```python
from build123d import *

# Parameters (mm, degrees)
F0_W     = 38.1
F0_H     = 38.1
F0_R     = 6.35
F1_DEPTH = 3.175
F2_W     = 38.1
F2_H     = 12.7
F3_DEPTH = 25.4
F4_W     = 38.1
F4_H     = 12.7
F5_DEPTH = 43.18
F6_R     = 3.175
F7_DEPTH = 81.281


with BuildPart() as f1:
    # F0 (on Top) → F1 (new body)
    with BuildSketch(Plane.XY):
        with Locations((19.05, 19.05)):
            Rectangle(F0_W, F0_H)
        with Locations((19.05, 25.4)):
            Circle(F0_R, mode=Mode.SUBTRACT)
    extrude(amount=F1_DEPTH)

    # F2 (on face) → F3 (join)
    with BuildSketch(Plane.XY.offset(3.175)):
        with Locations((19.05, 6.35)):
            Rectangle(F2_W, F2_H)
    extrude(amount=F3_DEPTH)

    # F4 (on face) → F5 (join)
    with BuildSketch(Plane.XZ):
        with Locations((19.05, 22.225)):
            Rectangle(F4_W, F4_H)
    extrude(amount=F5_DEPTH)

    # F6 (on face) → F7 (cut, through all)
    with BuildSketch(Plane.XZ.offset(43.18)):
        with Locations((19.05, 22.225)):
            Circle(F6_R)
    extrude(amount=-F7_DEPTH, mode=Mode.SUBTRACT)


solid = f1.part
```
The listing builds one solid part. Answer for the finished solid, in the listing's coordinates (mm). A direction names the side the tool comes from. Give positions to 0.01 mm unless a question says otherwise; leave off trailing zeros. Write each loop counter-clockwise with the first axis right and the second up, starting at its lowest first coordinate (ties: lowest second). Pieces come first, ordered by that corner, then holes. Notation, with made-up numbers: (-12.75, 26) -> (37.25, 26) arc R21 ccw to (37.25, 54) -> close; hole circle Ø10 at (-4.75, 81.5). An arc over 180 degrees is marked (long way). Write item = value, one per line. Start each with the question number.
1) The part is cut by section D-D, the plane x = 34.5. Determine the outline of the cut face in (y, z) (3 decimals).
2) Determine the mould class of faces 1 (the face through (23, -43.18, 22)), 2 (the face through (38.1, -11, 17)), 3 (the face through (0, -11, 17)), 4 (the face through (24.916, 22.968, 1.565)) for opening direction X: +X half, -X half, draft (parallel to the pull), parting line (faces both ways), or undercut.
3) Each of these flat-tipped pins is pushed along its axis until it touches: pin 1 (12.5 mm diameter, centred on x = 19, z = 18, fed in from +Y); pin 2 (20.5 mm diameter, centred on x = 16.5, y = 31.5, fed in from +Z) (3 decimals); pin 3 (10 mm diameter, centred on x = 13, y = -22, fed in from -Z) (3 decimals). Where does it stop, or does it pass through?
4) The part is cut by section B-B, the plane y = 25.4. Determine the outline of the cut face in (x, z) (3 decimals).
5) Straight lines are drawn through the part: line 1 along Y through (x, z) = (19.05, 2.3); line 2 along Y through (x, z) = (36, 18.5); line 3 along Y through (x, z) = (27.5, 3.25). For each, find the intervals that lie inside material, in ascending order.
6) Which of the six approach directions +Z, -Z, +X, -X, +Y, -Y give full straight-line access (tool end or side, diameter ignored) to faces 5 (the face through (19, -15, 28.575)), 6 (the face through (19, 12.7, 16)), 7 (the face through (19, 0, 8))?
7) The part is cut by section C-C, the plane z = 23.75. Determine the outline of the cut face in (x, y).
8) The part is cut by section A-A, the plane x = 19.05. Determine the outline of the cut face in (y, z) (3 decimals).
Solutions:
q1.outline = (-43.18, 15.875) -> (0, 15.875) -> (0, 0) -> (38.1, 0) -> (38.1, 3.175) -> (12.7, 3.175) -> (12.7, 28.575) -> (-43.18, 28.575) -> close
q2.face_1 = draft
q2.face_2 = +X half
q2.face_3 = -X half
q2.face_4 = undercut
q3.pin_1 = 12.7
q3.pin_2 = 3.175
q3.pin_3 = 15.875
q4.outline = (0, 0) -> (12.7, 0) -> (12.7, 3.175) -> (0, 3.175) -> close; (25.4, 0) -> (38.1, 0) -> (38.1, 3.175) -> (25.4, 3.175) -> close
q5.line_1 = 0 to 19.05, 31.75 to 38.1
q5.line_2 = -43.18 to 12.7
q5.line_3 = 0 to 12.7
q6.face_5 = +Z, +X, -X, +Y, -Y
q6.face_6 = +Z, +X, -X, +Y
q6.face_7 = -Z, +X, -X, -Y
q7.outline = (0, -43.18) -> (16.27, -43.18) -> (16.27, 12.7) -> (0, 12.7) -> close; (21.83, -43.18) -> (38.1, -43.18) -> (38.1, 12.7) -> (21.83, 12.7) -> close
q8.outline = (-43.18, 15.875) -> (0, 15.875) -> (0, 0) -> (19.05, 0) -> (19.05, 3.175) -> (12.7, 3.175) -> (12.7, 19.05) -> (-43.18, 19.05) -> close; (-43.18, 25.4) -> (12.7, 25.4) -> (12.7, 28.575) -> (-43.18, 28.575) -> close; (31.75, 0) -> (38.1, 0) -> (38.1, 3.175) -> (31.75, 3.175) -> close
